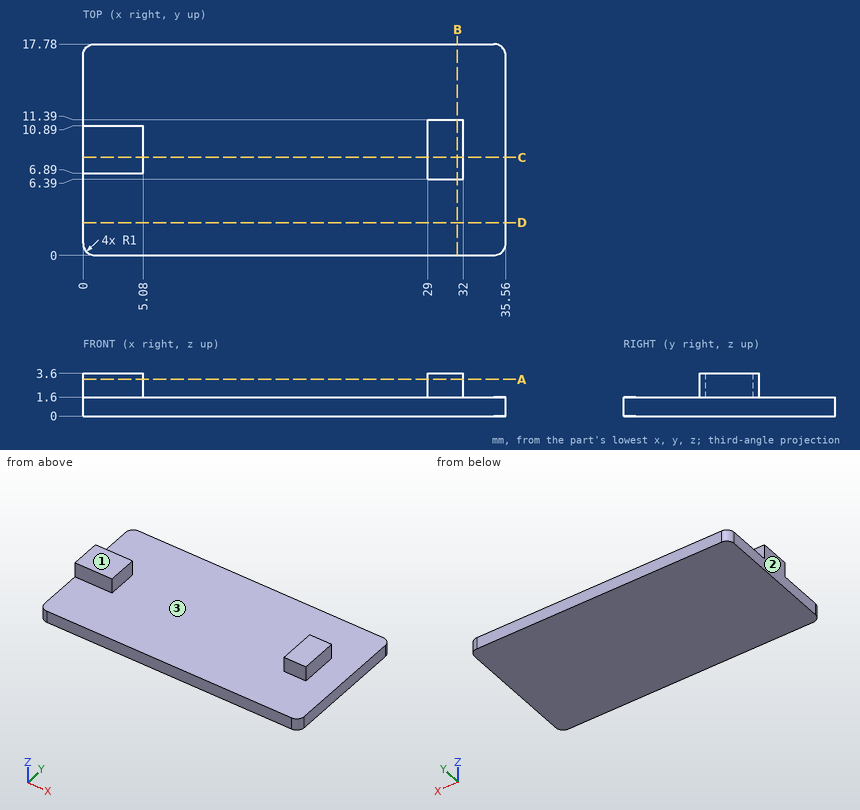
Geometry check sheet. Reference: drawing and pictorial views, mm from the part's lowest x, y, z. Give positions to 0.01 mm unless a question says otherwise; leave off trailing zeros. Order: outer loops, then holes, each group sorted by start corner. A loop starts at its lowest first (then second) coordinate and runs counter-clockwise, first axis right, second up. Notation, with made-up numbers: M 74.5,-23.75 L 133.5,-23.75 A12 ccw 133.5,-10.75 Z; hole C -29.75,86 d11. An arc over 180 degrees is marked long. Use one line per item in the form item = value. Start each with the question number.
Q1. Section check C-C (y = 8.25). Enter the section's corners in (x, z).
Q2. Mould release check, pull along X, two halves, no side actions. Record for the marked faces 1, 2 and 3: +X half, -X half, draft (parallel to the pull), parting line (faces both ways), or undercut.
Q3. Section check A-A (z = 3.1). Enter the section's corners in (x, y), then the cut area to 3 significant figures.
Q4. Section check B-B (x = 31.5). Enter the section's corners in (y, z).
Q5. Go/stop test with flat-tipped pins: pin 1 Ø1.6 at (x, z) = (1.5, 3) entering from +Y; pin 2 Ø8 at (x, y) = (30.5, 15.5) entering from +Z; pin 3 Ø1.6 at (y, z) = (10, 2.5) entering from +X. Record where each tip stops, or that it passes through.
Q6. Section check D-D (y = 2.75). Enter the section's corners in (x, z).
Q7. Scan lines: line 1 along X through (y, z) = (9.5, 1.8); line 2 along Z through (x, y) = (5.5, 4.5); line 3 along Y through (x, z) = (30, 3.35). Record each from-to range of solid material in increasing order. Write a range as [from, to].
Evaluation:
q1.outline = M 0,0 L 35.56,0 L 35.56,1.6 L 32,1.6 L 32,3.6 L 29,3.6 L 29,1.6 L 5.08,1.6 L 5.08,3.6 L 0,3.6 Z
q2.face_1 = draft
q2.face_2 = -X half
q2.face_3 = undercut
q3.outline = M 0,6.89 L 5.08,6.89 L 5.08,10.89 L 0,10.89 Z; M 29,6.39 L 32,6.39 L 32,11.39 L 29,11.39 Z
q3.area = 35.3 mm2
q4.outline = M 0,0 L 17.78,0 L 17.78,1.6 L 11.39,1.6 L 11.39,3.6 L 6.39,3.6 L 6.39,1.6 L 0,1.6 Z
q5.pin_1 = 10.89
q5.pin_2 = 1.6
q5.pin_3 = 32
q6.outline = M 0,0 L 35.56,0 L 35.56,1.6 L 0,1.6 Z
q7.line_1 = [0, 5.08], [29, 32]
q7.line_2 = [0, 1.6]
q7.line_3 = [6.39, 11.39]
